Check sheet for the modelled part. Datum: model origin and axes. Units: mm. A direction names the side the tool comes from. Coordinates: 2 decimals unless noted, no trailing zeros. Loops run counter-clockwise (first coordinate to the right, second up) from the corner with the lowest first, then second, coordinate; pieces in that order, holes last. Notation, with made-up numbers: (85.5, 59.5) -> (135.5, 59.5) arc R21 cw to (135.5, 80.5) -> close; hole circle Ø11 at (-14, 19.25). An arc over 180 degrees is marked (long way). Use one line per item in the form item = value.
from build123d import *

# Parameters (mm, degrees)
SKETCH_R     = 2.5
PAD_DEPTH    = 5
PAD001_DEPTH = 20


with BuildPart() as part:
    # Sketch → Pad (new body)
    with BuildSketch(Plane.XY):
        with BuildLine():
            ThreePointArc((0, 3.5), (-3.5, 0), (0, -3.5))
            Line((57.98, -3.5), (0, -3.5))
            ThreePointArc((57.98, -3.5), (61.48, 0), (57.98, 3.5))
            Line((0, 3.5), (57.98, 3.5))
        make_face()
        Circle(SKETCH_R, mode=Mode.SUBTRACT)
        with Locations((57.98, 0)):
            Circle(SKETCH_R, mode=Mode.SUBTRACT)
    extrude(amount=PAD_DEPTH)

    # Sketch001 (on Face8 of Pad) → Pad001 (join)
    with BuildSketch(Plane.XY.offset(5)):
        with BuildLine():
            Line((29.489935, 16), (29.489935, 6))
            Line((28.489935, 6), (29.489935, 6))
            Line((28.489935, 6), (28.489935, 15.99995))
            Line((9.108103, 11.918157), (28.489935, 15.99995))
            ThreePointArc((14.587373, -3.494502), (14.133535, 5.024439), (9.108103, 11.918157))
            Line((14.587373, -3.494502), (43.392665, -3.494502))
            ThreePointArc((49.388809, 12.296038), (43.956926, 5.32496), (43.392665, -3.494502))
            Line((29.489935, 16), (49.388809, 12.296038))
        make_face()
    extrude(amount=PAD001_DEPTH)


solid = part.part
(1) Section check C-C, the plane y = 14.5. Record the boundary of the cut face in (x, z).
Established:
outline = (21.37, 5) -> (28.49, 5) -> (28.49, 25) -> (21.37, 25) -> close; (29.49, 5) -> (37.55, 5) -> (37.55, 25) -> (29.49, 25) -> close
(2) Mould release check, pull along X, two halves, no side actions. Record for faces 6 (the flat face through (29, 4, 25)), 7 (the flat face through (29.49, 11, 15)), 8 (the flat face through (19, 14, 15)), 9 (the flat face through (39.3, 14.174, 14.86)): +X half, -X half, draft (parallel to the pull), parting line (faces both ways), or undercut.
Established:
face_6 = draft
face_7 = undercut
face_8 = -X half
face_9 = +X half
(3) Section check B-B, the plane z = 14.5. Record the boundary of the cut face in (x, y), plus the area to 3 significant figures.
Established:
outline = (9.11, 11.92) arc R15 cw to (14.59, -3.49) -> (43.39, -3.49) arc R15 cw to (49.39, 12.3) -> (29.49, 16) -> (29.49, 6) -> (28.49, 6) -> (28.49, 16) -> close
area = 552 mm²
(4) Scan lines: line 1 along Y through (x, z) = (57.98, 3.8); line 2 along Y through (x, z) = (33.5, 1.75); line 3 along Z through (x, y) = (51, -1.5). Record each from-to range of solid material in increasing order.
Established:
line_1 = -3.5 to -2.5, 2.5 to 3.5
line_2 = -3.5 to 3.5
line_3 = 0 to 5
(5) Section check A-A, the plane y = 0. Record the boundary of the cut face in (x, z).
Established:
outline = (-3.5, 0) -> (-2.5, 0) -> (-2.5, 5) -> (-3.5, 5) -> close; (2.5, 0) -> (55.48, 0) -> (55.48, 5) -> (42.98, 5) -> (42.98, 25) -> (15, 25) -> (15, 5) -> (2.5, 5) -> close; (60.48, 0) -> (61.48, 0) -> (61.48, 5) -> (60.48, 5) -> close
(6) Tool access check on faces 1 (the flat face through (29, 5.7, 5)), 2 (the cylindrical face through (14.174, 4.91, 14.86)), 3 (the cylindrical face through (44, 5.44, 14.86)), 4 (the flat face through (29, -3.5, 2)), 5 (the flat face through (28.49, 11, 15)). Record the directions out of +Z, -Z, +X, -X, +Y, -Y that give a thin tool (end or side, any length) a straight path to the whole face; none if there is none.
Established:
face_1 = -Z, +X, -X, +Y
face_2 = +Z, -X
face_3 = +Z, +X
face_4 = +Z, -Z, +X, -X, -Y
face_5 = +Z, -Z, +Y
(7) Section check D-D, the plane x = 53. Record the boundary of the cut face in (y, z), plus the area to 3 significant figures.
Established:
outline = (-3.5, 0) -> (3.5, 0) -> (3.5, 5) -> (-3.5, 5) -> close
area = 35.0 mm²
(8) Go/stop test with flat-tipped pins: P1, Ø3, axis at x = 16.5, y = 8.5, coming from the -Z side; P2, Ø6, axis at x = 47.5, z = 10.5, coming from the -Y side; P3, Ø8, axis at y = 10, z = 10.5, coming from the -X side. Record where each tip stops, or that it passes through.
Established:
P1 = 5
P2 = 6.58
P3 = 9.11
